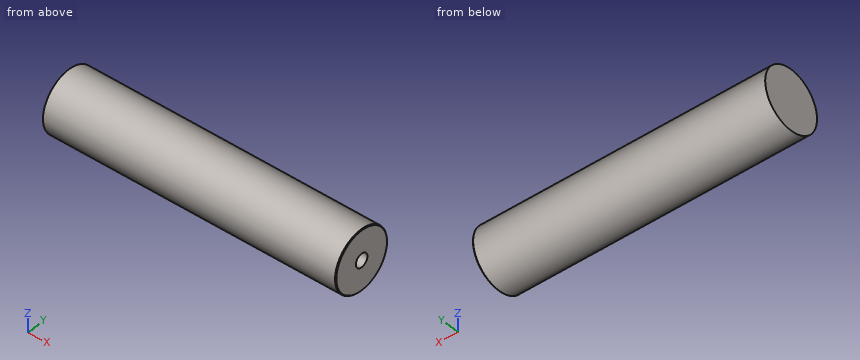
Autodesk Inventor part; units mm, degrees
ref_plane "YZ Plane" through (0, 0, 0) normal (1, 0, 0) x (0, 1, 0)
ref_plane "XZ Plane" through (0, 0, 0) normal (0, 1, 0) x (-1, 0, 0)
ref_plane "XY Plane" through (0, 0, 0) normal (0, 0, 1) x (1, 0, 0)
sketch "Sketch1" plane through (0, 0, 0) normal (1, 0, 0) x (0, 1, 0)
  circle A0 centre (0, 0) radius 11.1125
  dimension "d0" = 22.225
extrude "Extrusion1" add sketch "Sketch1" along normal blind 107.95
chamfer "Chamfer1" distance 0.254 angle 45 1 edges at (107.95, -11.1125, 0)
sketch "Sketch2" plane through (107.95, 0, 0) normal (1, 0, 0) x (0, 0, -1)
  circle A0 centre (0, 0) radius 11.1125
hole "Hole1" at (107.95, 0, 0) direction (-1, 0, 0) diameter 4.9784 depth 22.225 tip angle 118
properties material "Aluminum 6061"
Check sheet for the modelled part. Datum: model origin and axes. Units: mm. Coordinates: 2 decimals unless noted, no trailing zeros. Order: outer loops, then holes, each group sorted by start corner. A loop starts at its lowest first (then second) coordinate and runs counter-clockwise, first axis right, second up. Notation, with made-up numbers: M 10.5,76 L 49.5,76 A20 ccw 49.5,100 Z; hole C 55.25,21 d6. An arc over 180 degrees is marked long. Write each question's results on one line, items separated by ' | '. Start each with the question number.
1. Material ranges on probe 1 along Z at (x, y) = (102.25, 0); probe 2 along Y at (x, z) = (36.5, 0.25); probe 3 along Y at (x, z) = (35.5, 9.75), recorded low to high.
2. Go/stop test with flat-tipped pins: P1, Ø2, axis at x = 58.5, y = -3, coming from the -Z side; P2, Ø2, axis at x = 20, z = -4, coming from the +Y side; P3, Ø1.5, axis at x = 27, y = -2.5, coming from the -Z side. Record where each tip stops, or that it passes through.
3. Cross-section at A-A on x = 22. Record the cut outline in (y, z) (1 decimal), and give its area (3 significant figures).
Checks:
1) probe 1: z = -11.11 to -2.49, 2.49 to 11.11 | probe 2: y = -11.11 to 11.11 | probe 3: y = -5.33 to 5.33
2) P1: stops at z = -10.93 | P2: stops at y = 10.7 | P3: stops at z = -10.97
3) outline: C 0,0 d22.2 | area: 388 mm²
